Build history of the part. All positions in model axes, mm. Face numbers are marked on the shaded views. A direction names the side the tool comes from. Give positions to 0.01 mm unless a question says otherwise; leave off trailing zeros. Write each loop counter-clockwise with the first axis right and the second up, starting at its lowest first coordinate (ties: lowest second). Pieces come first, ordered by that corner, then holes. Notation, with made-up numbers: (-30.75, 52) -> (-9.75, 52) arc R14 ccw to (-9.75, 72) -> close; hole circle Ø10 at (75, 77.5). An arc over 180 degrees is marked (long way). Put each result on its own line as item: value.
Autodesk Inventor part; units mm, degrees
ref_plane "YZ Plane" through (0, 0, 0) normal (1, 0, 0) x (0, 1, 0)
ref_plane "XZ Plane" through (0, 0, 0) normal (0, 1, 0) x (-1, 0, 0)
ref_plane "XY Plane" through (0, 0, 0) normal (0, 0, 1) x (1, 0, 0)
sketch "Sketch1" plane through (0, 0, 0) normal (0, 1, 0) x (-1, 0, 0)
  circle A0 centre (0, 0) radius 5
  dimension "d0" = 10
extrude "Extrusion1" add sketch "Sketch1" along normal blind 15
sketch "Sketch2" plane through (0, 15, 0) normal (0, 1, 0) x (1, 0, 0)
  circle A0 centre (0, 0) radius 3.025
  dimension "d3" = 6.05
extrude "Extrusion2" cut sketch "Sketch2" against normal blind 12.5
sketch "Sketch3" plane through (0, 2.5, 0) normal (0, 1, 0) x (1, 0, 0)
  circle A0 centre (0, 0) radius 3.025 construction
  line L0 (-1.65, -3.3431) -> (-1.65, 4.0859) construction
  arc A1 (-1.65, 2.5354) -> (-1.65, -2.5354) centre (0, 0) ccw
  line L1 (-1.65, -2.5354) -> (-1.65, 2.5354)
  dimension "d6" = 1.65
extrude "Extrusion3" add sketch "Sketch3" along normal blind 10
sketch "Sketch4" plane through (0, 0, 0) normal (0, -1, 0) x (1, 0, 0)
  circle A0 centre (0, 0) radius 5
extrude "Extrusion4" cut sketch "Sketch4" against normal blind 8
properties part number "test_axis"
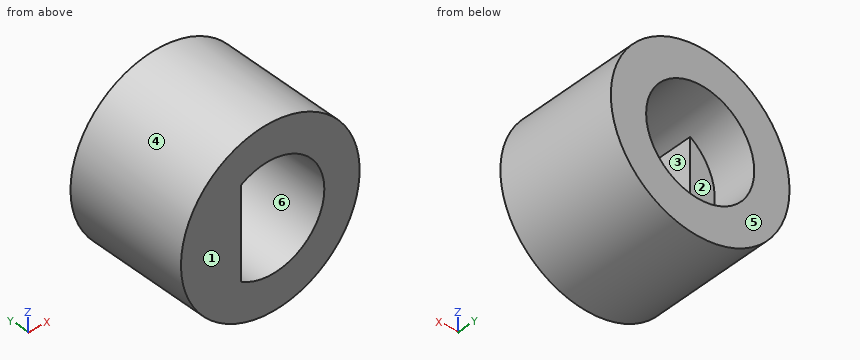
1) Slice it at C-C (y = 12). Write the cut outline in (x, z) (3 decimals), plus the area to 3 significant figures.
Filled sheet:
outline: circle Ø10 at (0, 0); hole (-1.65, -2.535) arc R3.025 ccw (long way) to (-1.65, 2.535) -> close
area: 54.7 mm2
2) Slice it at B-B (x = 0). Write the cut outline in (y, z) (3 decimals).
Filled sheet:
outline: (8, -5) -> (15, -5) -> (15, -3.025) -> (8, -3.025) -> close; (8, 3.025) -> (15, 3.025) -> (15, 5) -> (8, 5) -> close
3) Pull direction X, two halves, no side cores. Call the marked faces 3, 4, 5 and 6: released by +X, released by -X, zero draft, split by the parting line, or undercut.
Filled sheet:
face 3: undercut
face 4: split by the parting line
face 5: zero draft
face 6: undercut
4) Slice it at A-A (z = 0). Write the cut outline in (x, y) (3 decimals).
Filled sheet:
outline: (-5, 8) -> (-1.65, 8) -> (-1.65, 12.5) -> (-3.025, 12.5) -> (-3.025, 15) -> (-5, 15) -> close; (3.025, 8) -> (5, 8) -> (5, 15) -> (3.025, 15) -> close
5) Wall check: L1, parallel to Z at x = 0, y = 10.25 (3 decimals); L2, parallel to X at y = 11.75, z = 0 (3 decimals). Give the ranges that are in metal, low to high.
Filled sheet:
L1: -5 to -3.025, 3.025 to 5
L2: -5 to -1.65, 3.025 to 5
6) Pin check, flat tips, straight feed: pin 1 (1.5 mm diameter, centred on x = -2, z = -0.5, fed in from +Y); pin 2 (4 mm diameter, centred on x = -3, y = 9.5, fed in from -Z); pin 3 (1.5 mm diameter, centred on y = 11.5, z = 2.5, fed in from -X). Stop position of each tip, or through.
Filled sheet:
pin 1: y = 12.5
pin 2: z = -4.9
pin 3: x = -4.68
7) Tool access for the marked faces 1 and 2: list every direction of +Z, -Z, +X, -X, +Y, -Y with a clear straight run to the whole face (end or side of a thin tool).
Filled sheet:
face 1: +Z, -Z, +X, -X, -Y
face 2: +Y
8) Slice it at D-D (x = -1). Write the cut outline in (y, z), plus the area to 3 significant figures.
Filled sheet:
outline: (8, -4.9) -> (15, -4.9) -> (15, -2.85) -> (8, -2.85) -> close; (8, 2.85) -> (15, 2.85) -> (15, 4.9) -> (8, 4.9) -> close
area: 28.6 mm2
